Autodesk Inventor part; units mm, degrees
ref_plane "YZ Plane" through (0, 0, 0) normal (1, 0, 0) x (0, 1, 0)
ref_plane "XZ Plane" through (0, 0, 0) normal (0, 1, 0) x (-1, 0, 0)
ref_plane "XY Plane" through (0, 0, 0) normal (0, 0, 1) x (1, 0, 0)
sketch "スケッチ1" plane through (0, 0, 0) normal (1, 0, 0) x (0, 1, 0)
  line L0 (0, 0) -> (35.0104, -50)
  line L1 (35.0104, -50) -> (123, -50)
  line L2 (123, -50) -> (123, -40)
  line L3 (123, -40) -> (74.216, -40)
  line L4 (74.216, -40) -> (46.2077, 0)
  line L5 (46.2077, 0) -> (0, 0)
  line L6 (0, 10) -> (0, -60)
  point P0 (9.6049, -5)
  point P1 (43.6049, -5)
  dimension "d1" = 35
  dimension "d2" = 10
  dimension "d3" = 123
  dimension "d4" = 50
  dimension "d19" = 5
  dimension "d20" = 5
  dimension "d21" = 5
  dimension "d22" = 5
  dimension "d23" = 34
extrude "押し出し1" add sketch "スケッチ1" along normal mid plane 10
sketch "スケッチ2" plane through (5, 0, 0) normal (1, 0, 0) x (0, 0, -1)
  line L0 (0, 46.2077) -> (0, 0)
  line L1 (0, 0) -> (50, 35.0104)
  point P0 (5, 43.6049)
  point P1 (5, 9.6049)
  dimension "d9" = 5
  dimension "d10" = 5
  dimension "d11" = 34
hole "穴1" at (5, 43.6049, -5) at (5, 9.6049, -5) direction (-1, 0, 0) diameter 4.5 end through all
fillet "フィレット1" radius 5 4 edges at (0, 74.216, -40) (0, 46.2077, 0) (0, 0, 0) (0, 35.0104, -50)
fillet "フィレット2" radius 5 2 edges at (0, 123, -40) (0, 123, -50)
sketch "スケッチ3" plane through (5, 0, 0) normal (1, 0, 0) x (0, 0, -1)
  arc A0 (50, 118) -> (40, 118) centre (45, 118) ccw
  point P0 (0, 0)
hole "穴2" at (5, 118, -45) direction (-1, 0, 0) diameter 4 end through all
pattern_linear "矩形状パターン1" count 5 spacing 10 along (0, -1, 0) of "穴2"
sketch "スケッチ4" plane through (-5, 0, 0) normal (-1, 0, 0) x (0, 0, 1)
  line L0 (0, 36.6049) -> (-10, 36.6049)
  line L1 (-10, 36.6049) -> (-10, 16.6049)
  line L2 (-10, 16.6049) -> (0, 16.6049)
  line L3 (0, 16.6049) -> (0, 36.6049)
  line L4 (0, 9.6049) -> (0, 43.6049)
  circle A0 centre (-5, 43.6049) radius 2.25
  circle A1 centre (-5, 9.6049) radius 2.25
  point P0 (0, 0)
  dimension "d38" = 10
  dimension "d39" = 7
  dimension "d40" = 7
extrude "押し出し2" cut sketch "スケッチ4" against normal through all contours L3 L2 L1 L0
fillet "フィレット3" radius 3 4 edges at (0, 36.6049, 0) (0, 36.6049, -10) (0, 16.6049, -10) (0, 16.6049, 0)
properties part number "shooter_base8[" material "ABS プラスチック"
Can you work these out from the model? Positions are in its coordinate system, mm. A direction names the side the tool comes from. Coordinates: 2 decimals unless noted, no trailing zeros. Order: outer loops, then holes, each group sorted by start corner. A loop starts at its lowest first (then second) coordinate and runs counter-clockwise, first axis right, second up. Notation, with made-up numbers: (62, 88.5) -> (93, 88.5) arc R8 cw to (93, 95.5) -> close; hole circle Ø9 at (1, 48). An arc over 180 degrees is marked (long way). Use one line per item in the form item = value.
Q1. Imagine slicing it at D-D, the plane y = 103.5. List the corners of the cut face in (x, z) for me.
From the geometry:
outline = (-5, -50) -> (5, -50) -> (5, -40) -> (-5, -40) -> close
Q2. I need wall thicknesses on L1, parallel to Y at x = 0.75, z = -3; L2, parallel to Z at x = 1.5, y = 78; L3, parallel to Y at x = 3.25, z = -45. Which ranges of each line are inside material? Lowest first, please.
From the geometry:
L1 = 5.02 to 8.57, 10.64 to 16.6, 36.6 to 42.57, 44.64 to 48.31
L2 = -50 to -47, -43 to -40
L3 = 31.51 to 76, 80 to 86, 90 to 96, 100 to 106, 110 to 116, 120 to 123
Q3. Will these pins go through, and if not, where does the flat tip stop? P1, Ø3, axis at x = -1, z = -20.5, coming from the -Y side; P2, Ø5, axis at x = 1, y = 29, coming from the +Z side; P3, Ø3, axis at x = 0.5, z = -6, coming from the +Y side; P4, Ø4, axis at y = 43.6, z = -5, coming from the +X side.
From the geometry:
P1 = 13.3
P2 = -10
P3 = 51.46
P4 = through
Q4. We'd pull the mould along Y, two halves only. Please class faces 3 (the face through (0, 36.605, -5)), 4 (the face through (-0.07, 19.32, -27.59)), 5 (the face through (0, 12, 0)): released by +Y, released by -Y, zero draft, split by the parting line, or undercut.
From the geometry:
face_3 = undercut
face_4 = released by -Y
face_5 = zero draft
Q5. Imagine slicing it at A-A, the plane y = 88. List the corners of the cut face in (x, z) for me.
From the geometry:
outline = (-5, -50) -> (5, -50) -> (5, -47) -> (-5, -47) -> close; (-5, -43) -> (5, -43) -> (5, -40) -> (-5, -40) -> close
Q6. Which directions (+Z, -Z, +X, -X, +Y, -Y) give clear straight access to the entire face, cutting with the end or side of a thin tool? Please do faces 1 (the face through (-0.07, 45.884, -0.55)), 2 (the face through (0.07, 35.703, -9.145)).
From the geometry:
face_1 = +Z, +X, -X, +Y
face_2 = +Z, +X, -X
Q7. Imagine slicing it at B-B, the plane x = 3. Give the number of separate pieces and of enclosed holes in the cut face, then the cut area to 3 significant figures.
From the geometry:
separate_pieces = 1
enclosed_holes = 7
area = 2,440 mm²
Q8. Imagine slicing it at C-C, the plane z = -5. List the corners of the cut face in (x, y) for me.
From the geometry:
outline = (-5, 4.6) -> (5, 4.6) -> (5, 7.35) -> (-5, 7.35) -> close; (-5, 11.85) -> (5, 11.85) -> (5, 16.6) -> (-5, 16.6) -> close; (-5, 36.6) -> (5, 36.6) -> (5, 41.35) -> (-5, 41.35) -> close; (-5, 45.85) -> (5, 45.85) -> (5, 49.71) -> (-5, 49.71) -> close
